The figure shows three views and two pictorial views of one solid part (mm, origin at its lowest corner). Answer the questions. A direction names the side the tool comes from. Round coordinates to 2 decimals unless told otherwise and drop trailing zeros. Order: outer loops, then holes, each group sorted by start corner. A loop starts at its lowest first (then second) coordinate and runs counter-clockwise, first axis right, second up. Notation, with made-up numbers: (-23.5, 57) -> (9.5, 57) arc R25 cw to (9.5, 76) -> close; hole circle Ø10 at (29, -2). An arc over 180 degrees is marked (long way). Answer as a JSON object with one key per item and string values. Group by question number.
Item 1: For the marked faces 5 and 6, determine the directions among +Z, -Z, +X, -X, +Y, -Y from which every point of the face is accessible in a straight line to the end or side of a thin tool.
Item 2: The mould has two halves that part along X. Classify the marked faces 1, 2, 3 and 4: pulls with the +X half, pulls with the -X half, needs draft (parallel to the pull), parting line crosses it, or undercut.
Item 3: Given P1, Ø1, axis at x = 16, y = 7.5, coming from the -Z side, flat-ended and moving along its own axis, determine where the tip first touches the part or whether it passes through.
Item 4: Section A-A, the plane x = 10 is taken. Write down the section's boundary in (y, z), plus the area to 3 significant figures.
Item 5: Section D-D, the plane y = 3.75 is taken. Write down the section's boundary in (x, z).
Item 6: Section B-B, the plane y = 9 is taken. Write down the section's boundary in (x, z), plus the area to 3 significant figures.
Item 7: Consider probe 1 along X at (y, z) = (6, 5); probe 2 along Z at (x, y) = (10, 7); probe 3 along X at (y, z) = (7, 4.25). Determine where each line is inside the solid, lowest interval first. Write a range as from..to.
Item 8: Section C-C, the plane z = 7.25 is taken. Write down the section's boundary in (x, y).
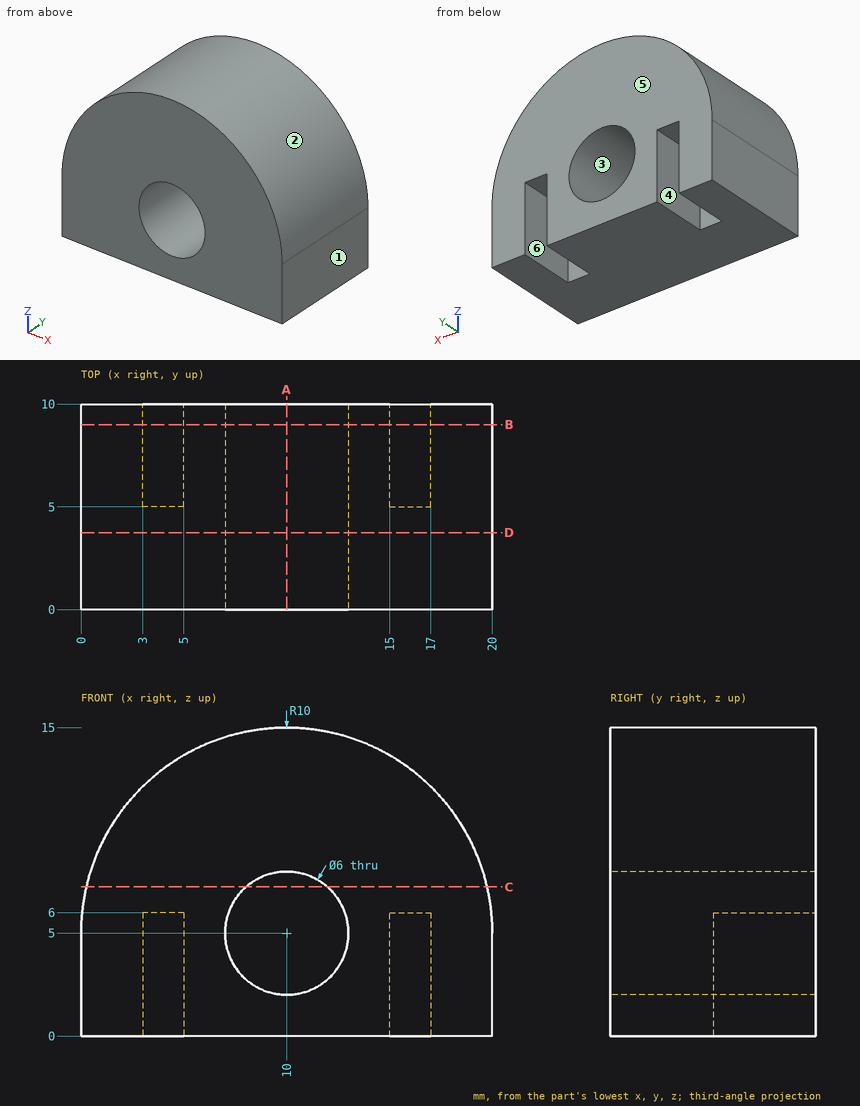
Values found:
{
 "1": {"face 5": "+Z, -Z, +X, -X, +Y", "face 6": "-Z, +Y"},
 "2": {"face 1": "pulls with the +X half", "face 2": "parting line crosses it", "face 3": "undercut", "face 4": "undercut"},
 "3": {"P1": "z = 6"},
 "4": {"outline": "(0, 0) -> (10, 0) -> (10, 2) -> (0, 2) -> close; (0, 8) -> (10, 8) -> (10, 15) -> (0, 15) -> close", "area": "90.0 mm2"},
 "5": {"outline": "(0, 0) -> (20, 0) -> (20, 5) arc R10 ccw to (0, 5) -> close; hole circle Ø6 at (10, 5)"},
 "6": {"outline": "(0, 0) -> (3, 0) -> (3, 6) -> (5, 6) -> (5, 0) -> (15, 0) -> (15, 6) -> (17, 6) -> (17, 0) -> (20, 0) -> (20, 5) arc R10 ccw to (0, 5) -> close; hole circle Ø6 at (10, 5)", "area": "205 mm2"},
 "7": {"probe 1": "0..3, 5..7, 13..15, 17..20", "probe 2": "0..2, 8..15", "probe 3": "0..3, 5..7.1, 12.9..15, 17..20"},
 "8": {"outline": "(0.26, 0) -> (8.02, 0) -> (8.02, 10) -> (0.26, 10) -> close; (11.98, 0) -> (19.74, 0) -> (19.74, 10) -> (11.98, 10) -> close"}
}
